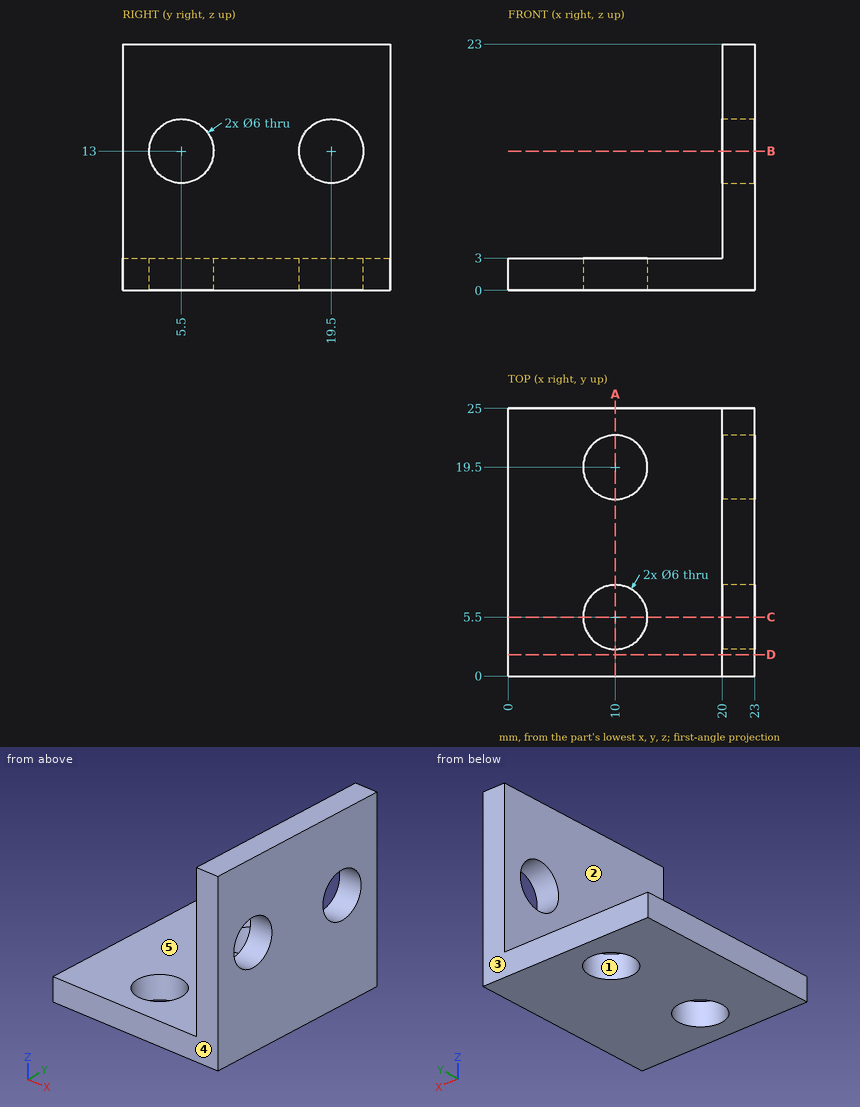
Part print with two shaded views. Sizes in mm from the minimum x, y, z corner. A direction names the side the tool comes from. Give positions to 0.01 mm unless a question says otherwise; leave off trailing zeros. Order: outer loops, then holes, each group sorted by start corner. A loop starts at its lowest first (then second) coordinate and runs counter-clockwise, first axis right, second up. Notation, with made-up numbers: M 70,-13.5 L 77,-13.5 A21 cw 77,3.5 Z; hole C 54.5,11 d8. An arc over 180 degrees is marked long. Put each result on its own line as item: value.
Item 1: Drop flat-ended pins along their axis: pin 1 Ø8 at (x, z) = (3, 9.5) entering from -Y; pin 2 Ø8 at (x, y) = (10, 19.5) entering from +Z; pin 3 Ø10 at (y, z) = (18, 8.5) entering from -X. Give the stop position or say it passes through.
Results are:
pin 1: through
pin 2: z = 3
pin 3: x = 20
Item 2: Cut at B-B on z = 13. Write the cut outline in (x, y).
Results are:
outline: M 20,0 L 23,0 L 23,2.5 L 20,2.5 Z; M 20,8.5 L 23,8.5 L 23,16.5 L 20,16.5 Z; M 20,22.5 L 23,22.5 L 23,25 L 20,25 Z
Item 3: Pull direction Y, two halves, no side cores. Call the marked faces 1, 2 and 3: +Y half, -Y half, draft (parallel to the pull), parting line (faces both ways), or undercut.
Results are:
face 1: undercut
face 2: draft
face 3: +Y half
Item 4: Which spindle directions (+Z, -Z, +X, -X, +Y, -Y) get a long thin tool onto all of the face, cutting with end or side? Do the marked faces 4 and 5. Say none if no direction does.
Results are:
face 4: +Z, -Z, +X, -X, -Y
face 5: +Z, -X, +Y, -Y
Item 5: Cut at D-D on y = 2. Write the cut outline in (x, z), then the cut area to 3 significant figures.
Results are:
outline: M 0,0 L 23,0 L 23,23 L 20,23 L 20,3 L 0,3 Z
area: 129 mm2
Item 6: Cut at A-A on x = 10. Write the cut outline in (y, z), then the cut area to 3 significant figures.
Results are:
outline: M 0,0 L 2.5,0 L 2.5,3 L 0,3 Z; M 8.5,0 L 16.5,0 L 16.5,3 L 8.5,3 Z; M 22.5,0 L 25,0 L 25,3 L 22.5,3 Z
area: 39.0 mm2
Item 7: Wall check: probe 1 along Y at (x, z) = (10, 1.3); probe 2 along X at (y, z) = (5.5, 1.35); probe 3 along Z at (x, y) = (21.7, 5.5). Give the ranges that are in metal, low to high.
Results are:
probe 1: 0 to 2.5, 8.5 to 16.5, 22.5 to 25
probe 2: 0 to 7, 13 to 23
probe 3: 0 to 10, 16 to 23
Item 8: Cut at C-C on y = 5.5. Write the cut outline in (x, z).
Results are:
outline: M 0,0 L 7,0 L 7,3 L 0,3 Z; M 13,0 L 23,0 L 23,10 L 20,10 L 20,3 L 13,3 Z; M 20,16 L 23,16 L 23,23 L 20,23 Z
